Work out the finished part from the listing and answer in its coordinate system (mm). Face numbers are marked on the shaded views. Give positions to 0.01 mm unless a question says otherwise; leave off trailing zeros. Loops run counter-clockwise (first coordinate to the right, second up) from the corner with the lowest first, then second, coordinate; pieces in that order, holes last. Notation, with made-up numbers: M -3,85 L 28,85 A23 ccw 28,99 Z; hole C 21,33.25 d5. An arc over 180 degrees is marked long. Use a Markdown table: item, result.
```python
from build123d import *

# Parameters (mm, degrees)
F1_DEPTH = 51.5
F2_DEPTH = 20
F3_DEPTH = 32
F5_DEPTH = 200.001


with BuildPart() as f1:
    # F0 (on Right) → F1 (new body, symmetric)
    with BuildSketch(Plane.YZ):
        Polygon((0, 3), (0, 0), (200, 0), (200, 63), (186.486487, 63), align=None)
        Polygon((0, 18), (0, 3), (186.486487, 63), (139.864865, 63), align=None)
        Polygon((0, 30), (0, 18), (139.864865, 63), (102.567568, 63), align=None)
    extrude(amount=F1_DEPTH, both=True)

    # F0 (on Right) → F2 (cut, symmetric)
    with BuildSketch(Plane.YZ):
        Polygon((0, 30), (0, 18), (139.864865, 63), (102.567568, 63), align=None)
    extrude(amount=F2_DEPTH, both=True, mode=Mode.SUBTRACT)

    # F0 (on Right) → F3 (cut, symmetric)
    with BuildSketch(Plane.YZ):
        Polygon((0, 18), (0, 3), (186.486487, 63), (139.864865, 63), align=None)
    extrude(amount=F3_DEPTH, both=True, mode=Mode.SUBTRACT)

    # F4 (on Front) → F5 (cut, through all)
    with BuildSketch(Plane.XZ):
        with BuildLine():
            Line((-51.5, 0), (0, 0))
            ThreePointArc((0, 0), (-25.76941, 0.500188), (-51.5, 2))
            Line((-51.5, 2), (-51.5, 0))
        make_face()
        with BuildLine():
            ThreePointArc((51.5, 2), (25.76941, 0.500188), (0, 0))
            Line((0, 0), (51.5, 0))
            Line((51.5, 0), (51.5, 2))
        make_face()
    extrude(amount=-F5_DEPTH, mode=Mode.SUBTRACT)


solid = f1.part
```
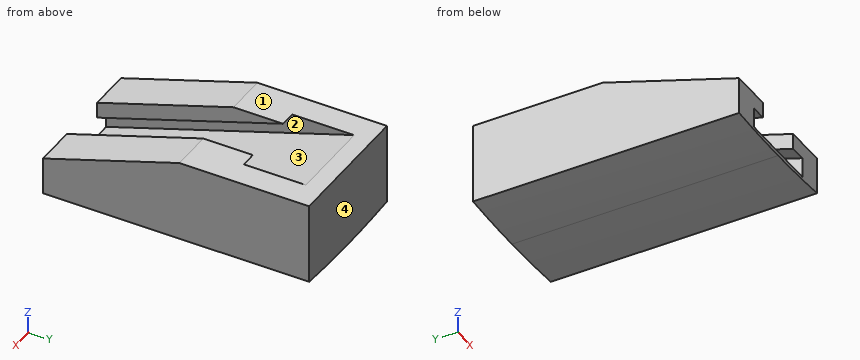
(1) A cutting plane is placed at A-A (z = 22.5). Write down the section's boundary in (x, y).
Entries:
| item | result |
|---|---|
| outline | M -51.5,0 L -20,0 L -20,13.99 L -32,13.99 L -32,60.61 L 32,60.61 L 32,13.99 L 20,13.99 L 20,0 L 51.5,0 L 51.5,200 L -51.5,200 Z |
(2) A cutting plane is placed at C-C (x = 11). Write down the section's boundary in (y, z), and give its area (3 significant figures).
Entries:
| item | result |
|---|---|
| outline | M 0,0.09 L 200,0.09 L 200,63 L 186.49,63 L 0,3 Z |
| area | 6,990 mm² |
(3) The mould has two halves that part along Z. Classify the marked faces 1, 2, 3 and 4: released by +Z, released by -Z, zero draft, split by the parting line, or undercut.
Entries:
| item | result |
|---|---|
| face 1 | released by +Z |
| face 2 | undercut |
| face 3 | undercut |
| face 4 | zero draft |
(4) Consider probe 1 along X at (y, z) = (43, 35.5); probe 2 along X at (y, z) = (100, 38.5); probe 3 along Z at (x, y) = (-28.5, 82). Determine where each line is inside the solid, lowest interval first. Write a range as [from, to].
Entries:
| item | result |
|---|---|
| probe 1 | x = [-51.5, -20], [20, 51.5] |
| probe 2 | x = [-51.5, -32], [32, 51.5] |
| probe 3 | z = [0.61, 29.38], [44.38, 56.38] |
(5) A cutting plane is placed at D-D (y = 67). Write down the section's boundary in (x, z).
Entries:
| item | result |
|---|---|
| outline | M -51.5,2 A664.06 ccw 0,0 A664.06 ccw 51.5,2 L 51.5,51.56 L 20,51.56 L 20,39.56 L 32,39.56 L 32,24.56 L -32,24.56 L -32,39.56 L -20,39.56 L -20,51.56 L -51.5,51.56 Z |
(6) A cutting plane is placed at B-B (y = 166.5). Write down the section's boundary in (x, z), and give its area (3 significant figures).
Entries:
| item | result |
|---|---|
| outline | M -51.5,2 A664.06 ccw 0,0 A664.06 ccw 51.5,2 L 51.5,63 L 32,63 L 32,56.57 L -32,56.57 L -32,63 L -51.5,63 Z |
| area | 6,010 mm² |
